Here's how the part is built. I have some questions about the finished solid (model axes, mm). Face numbers are marked on the shaded views. A direction names the side the tool comes from. Give positions to 0.01 mm unless a question says otherwise; leave off trailing zeros. Write each loop counter-clockwise with the first axis right and the second up, starting at its lowest first coordinate (ties: lowest second). Pieces come first, ordered by that corner, then holes. Notation, with made-up numbers: M 49.5,-30 L 82.5,-30 A17 cw 82.5,-11 Z; hole C 76.5,43.25 d4. An arc over 180 degrees is marked long. Answer as CSV lines item,"result". Start each with the question number.
Q1. Suppose I cut it at C-C (z = 3.5). Write out the boundary of the cut face in (x, y), then the cut area to 3 significant figures.
Q2. Suppose I cut it at D-D (y = -6). Write out the boundary of the cut face in (x, z), then the cut area to 3 significant figures.
Q3. For pin 1 (6 mm diameter, centred on x = 1.5, y = -5, fed in from +Z); pin 2 (1.8 mm diameter, centred on y = 0, z = -7.25, fed in from +X); pin 3 (4 mm diameter, centred on x = 1, y = 4.5, fed in from -Z); pin 4 (5 mm diameter, centred on x = -1.5, z = -6.5, fed in from +Y), each with a flat end and sliding along its axis, tell me the tip position at first contact or that it passes through.
Q4. Suppose I cut it at B-B (z = -7.75). Write out the boundary of the cut face in (x, y), then the cut area to 3 significant figures.
Q5. If I drill on line 1 along Z through (x, y) = (-2, 0); line 2 along X through (y, z) = (-5.5, 0); line 3 along Z through (x, y) = (2, -5.25), over which ranges is the centre line in solid material (lowest first)?
Q6. On a 3-axis mill with a long thin cutter (end or side, diameter ignored), from which of +Z, -Z, +X, -X, +Y, -Y can I reach the whole of each face in a straight line? I mean the marked faces 4 and 5. Say none if no direction works.
Q7. Suppose I cut it at A-A (y = 5.75). Write out the boundary of the cut face in (x, z).
Q8. Thinking about a two-plate mould opening in Y: for the marked faces 1, 2 and 3, which applies, +Y half, -Y half, draft (parallel to the pull), parting line (faces both ways), or undercut?
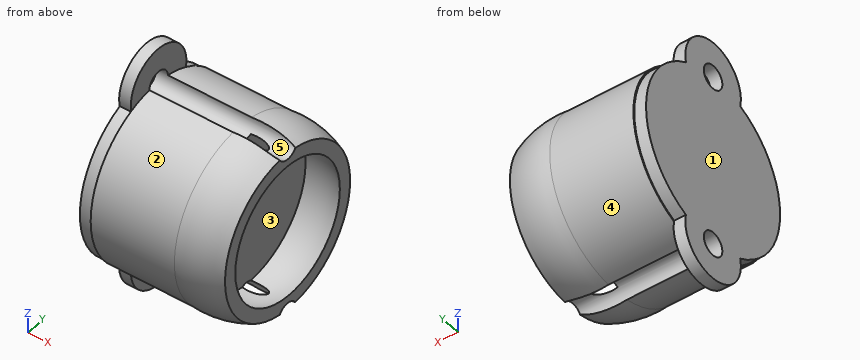
```python
from build123d import *
from build123d.topology import SkipClean

# Parameters (mm, degrees)
ENL_V_START             = 3
ESQUISSE2_W             = 20.168692272
ESQUISSE2_H             = 19.901202985
ENL_V_MAT_EXTRU_1_DEPTH = 10
BOSS_EXTRU_1_START      = -11
ESQUISSE3_R             = 7.25
BOSS_EXTRU_1_DEPTH      = 1
ESQUISSE4_R             = 7.35
BOSS_EXTRU_2_DEPTH      = 7.5
ESQUISSE5_R             = 3
ESQUISSE5_R_2           = 1
BOSS_EXTRU_3_DEPTH      = 1
ESQUISSE6_R             = 1
ENL_V_MAT_EXTRU_2_DEPTH = 18.430504869


with BuildPart() as part:
    # Esquisse1 → R_volution1 (revolve)
    with SkipClean():  # the faces are left unmerged after this step: merging them gives an invalid solid
        with BuildSketch(Plane.XY):
            with BuildLine():
                ThreePointArc((-6.4, 0), (0, 6.4), (6.4, 0))
                Line((6.4, 0), (7.4, 0))
                ThreePointArc((7.4, 0), (0, 7.4), (-7.4, 0))
                Line((-7.4, 0), (-6.4, 0))
            make_face()
            with BuildLine():
                Line((7.4, 0), (6.4, 0))
                ThreePointArc((6.4, 0), (0, -6.4), (-6.4, 0))
                Line((-6.4, 0), (-7.4, 0))
                ThreePointArc((-7.4, 0), (0, -7.4), (7.4, 0))
            make_face()
        revolve(axis=Axis((-7.4, 0, 0), (1, 0, 0)))
    add(part.part.scale(1), mode=Mode.REPLACE)  # the faces are merged on a copy

    # Esquisse2 → Enl_v. mat.-Extru.1 (cut)
    with BuildSketch(Plane(origin=(0, 0, 0), x_dir=(0, 0, -1), z_dir=(1, 0, 0)).offset(ENL_V_START)):
        with Locations((-0.294238216, 0.080246787)):
            Rectangle(ESQUISSE2_W, ESQUISSE2_H)
    extrude(amount=ENL_V_MAT_EXTRU_1_DEPTH, mode=Mode.SUBTRACT)



with BuildPart() as body_2:
    # Esquisse3 → Boss.-Extru.1 (new body)
    with BuildSketch(Plane(origin=(3, 0, 0), x_dir=(0, 0, -1), z_dir=(1, 0, 0)).offset(BOSS_EXTRU_1_START)):
        Circle(ESQUISSE3_R)
    extrude(amount=-BOSS_EXTRU_1_DEPTH)


with BuildPart() as part_1:
    add(part.part)

    add(body_2.part)  # Boss.-Extru.2 merges body 2
    # Esquisse4 → Boss.-Extru.2 (add)
    with BuildSketch(Plane(origin=(-8, 0, 0), x_dir=(0, 0, -1), z_dir=(1, 0, 0))):
        with Locations(Location((0, 0, 0), (0, 0, 90))):
            Circle(ESQUISSE4_R)
    extrude(amount=BOSS_EXTRU_2_DEPTH)

    # Esquisse5 → Boss.-Extru.3 (add)
    # profile 1 of 2: a face of its own
    with BuildSketch(Plane.ZY.offset(9)):
        with Locations((7.25, 0)):
            Circle(ESQUISSE5_R)
        with Locations((7.25, 0)):
            Circle(ESQUISSE5_R_2, mode=Mode.SUBTRACT)
    # profile 2 of 2: a face of its own
    with BuildSketch(Plane.ZY.offset(9)):
        with Locations((-7.25, 0)):
            Circle(ESQUISSE5_R)
        with Locations((-7.25, 0)):
            Circle(ESQUISSE5_R_2, mode=Mode.SUBTRACT)
    extrude(amount=-BOSS_EXTRU_3_DEPTH)

    # Esquisse6 → Enl_v. mat.-Extru.2 (cut, through all)
    with BuildSketch(Plane.ZY.offset(9)):
        with Locations((-7.25, 0)):
            Circle(ESQUISSE6_R)
        with Locations((7.25, 0)):
            Circle(ESQUISSE6_R)
    extrude(amount=-ENL_V_MAT_EXTRU_2_DEPTH, mode=Mode.SUBTRACT)


solid = part_1.part
```
Resolved:
1,outline,"M -9,-6.35 L -8,-6.35 L -8,-6.46 L -0.86,-6.46 A6.52 ccw 3,-5.79 L 3,-4.44 A5.36 cw -0.5,-5.33 L -0.5,5.33 A5.36 cw 3,4.44 L 3,5.79 A6.52 ccw -0.86,6.46 L -8,6.46 L -8,6.35 L -9,6.35 Z"
1,area,"118 mm^2"
2,outline,"M -9,-4.07 L -8,-4.07 L -8,-4.25 L -0.86,-4.25 A4.33 ccw 3,-3.12 L 3,3.12 A4.33 ccw -0.86,4.25 L -8,4.25 L -8,4.07 L -9,4.07 Z; hole M -0.5,-2.17 A2.23 ccw long -0.5,2.17 Z"
2,area,"89.9 mm^2"
3,pin 1,"z = 7.06"
3,pin 2,"through"
3,pin 3,"z = -6.92"
3,pin 4,"y = 6.17"
4,outline,"M -9,-2.96 L -8,-2.96 L -8,-0.87 L -9,-0.87 Z; M -9,0.87 L -8,0.87 L -8,2.96 L -9,2.96 Z"
4,area,"4.18 mm^2"
5,line 1,"-6.25 to 6.25"
5,line 2,"-9 to -0.5"
5,line 3,"-4.82 to -3.07, 3.07 to 4.82"
6,face 4,"+Y"
6,face 5,"+X, -X"
7,outline,"M -9,-4.42 L -8,-4.42 L -8,-4.58 L -0.86,-4.58 A4.66 ccw 3,-3.56 L 3,3.56 A4.66 ccw -0.86,4.58 L -8,4.58 L -8,4.42 L -9,4.42 Z; hole M -0.5,-2.77 A2.81 ccw long -0.5,2.77 Z"
8,face 1,"draft"
8,face 2,"-Y half"
8,face 3,"undercut"
